Part model, mm, in its own coordinate system. Face numbers are marked on the shaded views. A direction names the side the tool comes from. Round coordinates to 2 decimals unless told otherwise and drop trailing zeros. Order: outer loops, then holes, each group sorted by start corner. A loop starts at its lowest first (then second) coordinate and runs counter-clockwise, first axis right, second up. Notation, with made-up numbers: (-0.5, 85.5) -> (33.5, 85.5) arc R11 cw to (33.5, 99.5) -> close; hole circle Ø3 at (-26, 83). An arc over 180 degrees is marked (long way). Use CSV: the item, a comma, the result in double quotes.
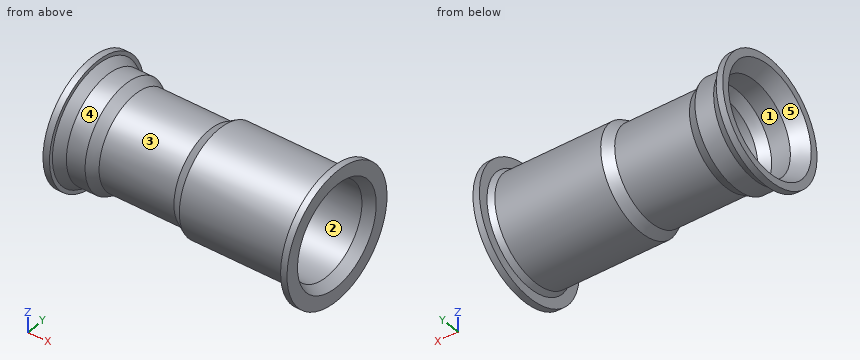
```python
from build123d import *


with BuildPart() as f1:
    # F0 (on Front) → F1 (revolve)
    with BuildSketch(Plane.XZ):
        Polygon((-105.55408, 62), (-105.55408, 66), (-112.55408, 66), (-112.55408, 57.958548), (-97.03742, 49), (-77.03742, 49), (-66.645115, 43), (17.106174, 43), (27.498479, 49), (140.737355, 49), (151.378544, 55.143693), (151.532518, 70), (144.673228, 70), (144.673228, 66), (144.673228, 59.355281), (138.86171, 56), (25.622834, 56), (15.23053, 50), (-64.76947, 50), (-75.161775, 56), (-95.161775, 56), align=None)
    revolve(axis=Axis((50.378699, 0, 0), (1, 0, 0)))


solid = f1.part
```
(1) Drop flat-ended pins along their axis: P1, Ø12, axis at x = 116.5, z = -32, coming from the +Y side; P2, Ø1.5, axis at x = 50.5, y = 48.5, coming from the +Z side; P3, Ø2, axis at x = -76.5, z = 31.5, coming from the +Y side. Give the stop position or say it passes through.
Reply:
P1,"y = 49.6"
P2,"z = 29.26"
P3,"y = 46.97"
(2) Cut at A-A, the plane x = -31. Give the cut face in (y, z).
Reply:
outline,"circle Ø100 at (0, 0); hole circle Ø86 at (0, 0)"
(3) Which spindle directions (+Z, -Z, +X, -X, +Y, -Y) get a long thin tool onto all of the face, cutting with end or side? Do the marked faces 4 and 5. Say none if no direction does.
Reply:
face 4,"none"
face 5,"-X"
(4) Probe probe 1 along Y at (x, z) = (-87.5, 0); probe 2 along Z at (x, y) = (-15, 0). List the from-to ranges inside material, lowest first. Write a range as [from, to].
Reply:
probe 1,"[-56, -49], [49, 56]"
probe 2,"[-50, -43], [43, 50]"
(5) Pull direction Z, two halves, no side cores. Call the marked faces 1, 2 and 3: released by +Z, released by -Z, zero draft, split by the parting line, or undercut.
Reply:
face 1,"undercut"
face 2,"undercut"
face 3,"split by the parting line"
(6) Cut at B-B, the plane x = 113.5. Give the cut face in (y, z), then the cut area to 3 significant figures.
Reply:
outline,"circle Ø112 at (0, 0); hole circle Ø98 at (0, 0)"
area,"2,310 mm2"
